Geometry check sheet. Reference: the model listing, model coordinates, mm. A direction names the side the tool comes from. Give positions to 0.01 mm unless a question says otherwise; leave off trailing zeros. Write each loop counter-clockwise with the first axis right and the second up, starting at its lowest first coordinate (ties: lowest second). Pieces come first, ordered by that corner, then holes. Notation, with made-up numbers: (42.25, -16.5) -> (92.25, -16.5) arc R10 ccw to (92.25, -8.5) -> close; hole circle Ø4 at (-6.5, -13). An arc over 180 degrees is marked (long way). Write item = value, one per line. Start each with the question number.
1. Depth check by flat-ended pin: P1, Ø0.9, axis at x = 22.5, y = 2, coming from the +Z side; P2, Ø8, axis at x = 17.5, z = 10, coming from the +Y side; P3, Ø3, axis at x = 34.5, z = 10.5, coming from the -Y side. Enter the tip coordinate at first touch or a pass-through.
2. Cross-section at C-C, the plane z = 15.25. Record the cut outline in (x, y), plus the area to 3 significant figures.
3. Cross-section at B-B, the plane z = 5.25. Record the cut outline in (x, y).
4. Set-up check for faces 1 (the flat face through (24, 16, 0)), 2 (the cylindrical face through (19.02, 2.61, 6.12)): record each of +Z, -Z, +X, -X, +Y, -Y from which the full face is reachable in a straight line by a thin tool's end or side.
5. Mould release check, pull along Y, two halves, no side actions. Record for faces 3 (the flat face through (11.74, 24.53, 0.59)), 4 (the cylindrical face through (43.74, 17.677, 0.587)), 5 (the flat face through (12.033, 6.684, 0.587)): pulls with the +Y half, pulls with the -Y half, needs draft (parallel to the pull), parting line crosses it, or undercut.
6. Thickness scan on line 1 along Z through (x, y) = (42, 19); line 2 along Y through (x, z) = (4, 0.7); line 3 along X through (y, z) = (6.5, 8.5). Record the ranges inside material, lowest first.
7. Cross-section at A-A, the plane x = 45. Record the cut outline in (y, z).
```python
from build123d import *

# Parameters (mm, degrees)
ESQUISSE1_R        = 2
BOSS_EXTRU_1_DEPTH = 1.19
ESQUISSE2_R        = 14
BOSS_EXTRU_2_DEPTH = 15
CONG_1_R           = 5
ESQUISSE3_R        = 9
BOSS_EXTRU_3_DEPTH = 9
CONG_2_R           = 8.9


with BuildPart() as part:
    # Esquisse1 → Boss.-Extru.1 (new body)
    with BuildSketch(Plane.XY):
        with BuildLine():
            Line((1.31508183, 18.266068418), (22.45508183, 30.966068418))
            ThreePointArc((22.45508183, 30.966068418), (24, 31.394448725), (25.54491817, 30.966068418))
            Line((25.54491817, 30.966068418), (46.68491817, 18.266068418))
            ThreePointArc((46.68491817, 18.266068418), (48.14, 15.694448725), (46.68491817, 13.122829031))
            Line((46.68491817, 13.122829031), (25.54491817, 0.422829031))
            ThreePointArc((25.54491817, 0.422829031), (24, -0.005551275), (22.45508183, 0.422829031))
            Line((22.45508183, 0.422829031), (1.31508183, 13.122829031))
            ThreePointArc((1.31508183, 13.122829031), (-0.14, 15.694448725), (1.31508183, 18.266068418))
        make_face()
        with Locations((44, 15.694448725)):
            Circle(ESQUISSE1_R, mode=Mode.SUBTRACT)
        with Locations(Location((4, 15.694448725, 0), (0, 0, 180))):
            Circle(ESQUISSE1_R, mode=Mode.SUBTRACT)
    extrude(amount=BOSS_EXTRU_1_DEPTH)

    # Esquisse2 → Boss.-Extru.2 (add)
    with BuildSketch(Plane.XY.offset(1.19)):
        with Locations(Location((24, 15.694448725, 0), (0, 0, 231.704406007))):
            Circle(ESQUISSE2_R)
    extrude(amount=BOSS_EXTRU_2_DEPTH)

    # Congé1
    cong_1_edges = [part.edges().sort_by_distance(p)[0] for p in [
        (32.676061537, 26.681985128, 16.19),
    ]]
    fillet(cong_1_edges, radius=CONG_1_R)

    # Esquisse3 → Boss.-Extru.3 (add)
    with BuildSketch(Plane.XY.offset(16.19)):
        with Locations((24, 15.694448725)):
            Circle(ESQUISSE3_R)
    extrude(amount=BOSS_EXTRU_3_DEPTH)

    # Congé2
    cong_2_edges = [part.edges().sort_by_distance(p)[0] for p in [
        (15, 15.694448725, 25.19),
    ]]
    fillet(cong_2_edges, radius=CONG_2_R)


solid = part.part
```
Answers:
q1.P1 = 13.7
q1.P2 = 29.47
q1.P3 = 4.97
q2.outline = circle Ø23.84 at (24, 15.69)
q2.area = 446 mm^2
q3.outline = circle Ø28 at (24, 15.69)
q4.face_1 = -Z, +X, -X, +Y, -Y
q4.face_2 = +Z
q5.face_3 = pulls with the +Y half
q5.face_4 = undercut
q5.face_5 = pulls with the -Y half
q6.line_1 = 0 to 1.19
q6.line_2 = 11.51 to 13.69, 17.69 to 19.88
q6.line_3 = 13.44 to 34.56
q7.outline = (12.11, 0) -> (13.96, 0) -> (13.96, 1.19) -> (12.11, 1.19) -> close; (17.43, 0) -> (19.28, 0) -> (19.28, 1.19) -> (17.43, 1.19) -> close
